Model file for the job. Use its own axes, mm. Face numbers are marked on the shaded views. A direction names the side the tool comes from. Round coordinates to 2 decimals unless told otherwise and drop trailing zeros. Order: outer loops, then holes, each group sorted by start corner. A loop starts at its lowest first (then second) coordinate and runs counter-clockwise, first axis right, second up. Notation, with made-up numbers: (8.5, 29.5) - (47.5, 29.5) arc R31 ccw to (47.5, 54.5) - close; hole circle Ø7 at (20, 64). An arc over 180 degrees is marked (long way). Put each result on its own line as item: value. Start each with the question number.
Item 1: Saw through at B-B on x = 0. List the corners of the cut face in (y, z).
Item 2: Which spindle directions (+Z, -Z, +X, -X, +Y, -Y) get a long thin tool onto all of the face, cutting with end or side? Do the marked faces 3 and 4. Say none if no direction does.
Item 3: Saw through at A-A on z = 2.45. List the corners of the cut face in (x, y).
Item 4: Saw through at C-C on y = 1. List the corners of the cut face in (x, z).
Item 5: Saw through at D-D on y = 4.5. List the corners of the cut face in (x, z).
Item 6: Probe probe 1 along Y at (x, z) = (38, 2.1); probe 2 along X at (y, z) = (0.5, 1.55); probe 3 along X at (y, z) = (1, 1.2). List the from-to ranges inside material, lowest first.
Item 7: Mould opens along X. For the marked faces 1 and 2 say: pulls with the +X half, pulls with the -X half, needs draft (parallel to the pull), parting line crosses it, or undercut.
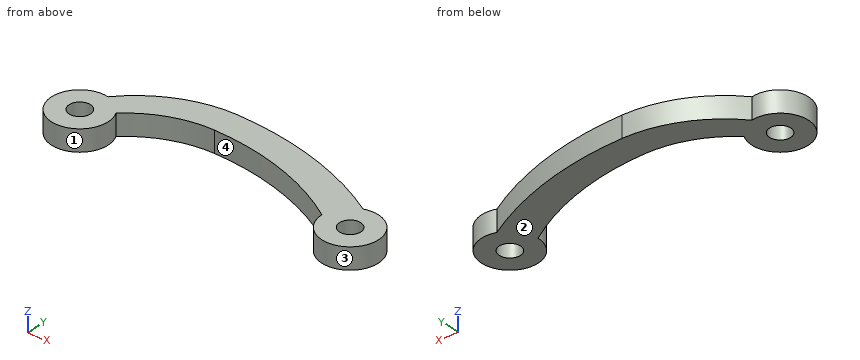
```python
from build123d import *

# Parameters (mm, degrees)
CROQUIS1_R              = 1.5
SALIENTE_EXTRUIR1_DEPTH = 3


with BuildPart() as part:
    # Croquis1 → Saliente-Extruir1 (new body)
    with BuildSketch(Plane.XY):
        with BuildLine():
            ThreePointArc((14, 6), (24.435686691, 4.476369784), (34.000133515, 0.032681824))
            ThreePointArc((34.000133515, 0.032681824), (41.241241669, -2.344003507), (36.716180593, 3.788377981))
            ThreePointArc((36.716180593, 3.788377981), (25.775070157, 8.419103062), (14, 10))
            ThreePointArc((14, 10), (6.711840205, 8.410145405), (0.74792205, 3.929454492))
            ThreePointArc((0.74792205, 3.929454492), (-2.369034826, -3.222991466), (3.52713505, 1.886615578))
            ThreePointArc((3.52713505, 1.886615578), (8.37414825, 4.934787082), (14, 6))
        make_face()
        Circle(CROQUIS1_R, mode=Mode.SUBTRACT)
        with Locations((38, 0)):
            Circle(CROQUIS1_R, mode=Mode.SUBTRACT)
    extrude(amount=SALIENTE_EXTRUIR1_DEPTH)


solid = part.part
```
Results found:
1. outline: (-4, 0) - (-1.5, 0) - (-1.5, 3) - (-4, 3) - close; (1.5, 0) - (4, 0) - (4, 3) - (1.5, 3) - close
2. face 3: +Z, -Z
2. face 4: +Z, -Z, -Y
3. outline: (0.75, 3.93) arc R4 ccw (long way) to (3.53, 1.89) arc R15.39 cw to (14, 6) arc R36.5 cw to (34, 0.03) arc R4 ccw (long way) to (36.72, 3.79) arc R44.64 ccw to (14, 10) arc R17.5 ccw to start; hole circle Ø3 at (0, 0); hole circle Ø3 at (38, 0)
4. outline: (-3.87, 0) - (-1.12, 0) - (-1.12, 3) - (-3.87, 3) - close; (1.12, 0) - (3.87, 0) - (3.87, 3) - (1.12, 3) - close; (32.44, 0) - (36.88, 0) - (36.88, 3) - (32.44, 3) - close; (39.12, 0) - (41.87, 0) - (41.87, 3) - (39.12, 3) - close
5. outline: (1.26, 0) - (7.37, 0) - (7.37, 3) - (1.26, 3) - close; (24.36, 0) - (35.47, 0) - (35.47, 3) - (24.36, 3) - close
6. probe 1: y = -4 to -1.5, 1.5 to 4
6. probe 2: x = -3.97 to -1.41, 1.41 to 3.97, 33.27 to 36.59, 39.41 to 41.97
6. probe 3: x = -3.87 to -1.12, 1.12 to 3.87, 32.44 to 36.88, 39.12 to 41.87
7. face 1: undercut
7. face 2: needs draft
